Part model, mm, in its own coordinate system. A direction names the side the tool comes from. Round coordinates to 2 decimals unless told otherwise and drop trailing zeros. Loops run counter-clockwise (first coordinate to the right, second up) from the corner with the lowest first, then second, coordinate; pieces in that order, holes last. Notation, with made-up numbers: M -31,24 L 21,24 A17 cw 21,31 Z; hole C -14.5,75.5 d3. An arc over 180 degrees is marked long. Put each result on its own line as item: value. Start each with the question number.
```python
from build123d import *

# Parameters (mm, degrees)
SKETCH_1_W          = 18
SKETCH_1_H          = 5
EXTRUDE_1_DEPTH     = 47.5
SKETCH_2_W          = 24
SKETCH_2_H          = 8
EXTRUDE_2_DEPTH     = 3.5
SKETCH_3_W          = 12.6
SKETCH_3_H          = 2
CUT_EXTRUDE_1_DEPTH = 50.30010142
CHAMFER_1_SIZE      = 1


with BuildPart() as part:
    # 草图1 → 凸台-拉伸1 (new body)
    with BuildSketch(Plane.XY):
        Rectangle(SKETCH_1_W, SKETCH_1_H)
    extrude(amount=EXTRUDE_1_DEPTH)

    # 草图2 → 凸台-拉伸2 (add)
    with BuildSketch(Plane(origin=(0, 0, 0), x_dir=(-1, 0, 0), z_dir=(0, 0, -1))):
        with Locations((0, 1.5)):
            Rectangle(SKETCH_2_W, SKETCH_2_H)
    extrude(amount=-EXTRUDE_2_DEPTH)

    # 草图3 → 切除-拉伸1 (cut, through all)
    with BuildSketch(Plane(origin=(0, 0, 0), x_dir=(-1, 0, 0), z_dir=(0, 0, -1))):
        with Locations((0, -1.5)):
            Rectangle(SKETCH_3_W, SKETCH_3_H)
    extrude(amount=-CUT_EXTRUDE_1_DEPTH, mode=Mode.SUBTRACT)

    # 倒角1
    chamfer_1_edges = [part.edges().sort_by_distance(p)[0] for p in [
        (12, 5.5, 1.75),
        (-12, 5.5, 1.75),
    ]]
    chamfer(chamfer_1_edges, length=CHAMFER_1_SIZE)


solid = part.part
```
1. Cut at B-B, the plane z = 20.5. Give the cut face in (x, y).
2. Which spindle directions (+Z, -Z, +X, -X, +Y, -Y) get a long thin tool onto all of the face, cutting with end or side? Do faces 1 (the flat face through (9, 0, 25)), 2 (the flat face through (0, 2.5, 25)), 3 (the flat face through (-9, 0, 25)), 4 (the flat face through (6.3, -2, 23)). Say none if no direction does.
3. Cut at D-D, the plane x = -8.25. Give the cut face in (y, z), and give its area (3 significant figures).
4. Drop flat-ended pins along their axis: pin 1 (3 mm diameter, centred on x = -5, y = 4.5, fed in from +Z); pin 2 (6.5 mm diameter, centred on x = -0.5, z = 28, fed in from -Y); pin 3 (2.5 mm diameter, centred on y = 1, z = 29, fed in from +X). Give the stop position or say it passes through.
5. Cut at C-C, the plane x = -1. Give the cut face in (y, z), and give its area (3 significant figures).
6. Wall check: L1, parallel to X at y = -1.5, z = 8; L2, parallel to Z at x = -9.25, y = -0.75; L3, parallel to Y at x = 7, z = 38.5. Give the ranges that are in metal, low to high.
7. Cut at A-A, the plane y = 0.5. Give the cut face in (x, z), and give its area (3 significant figures).
Results list:
1. outline: M -9,-2.5 L -6.3,-2.5 L -6.3,-0.5 L 6.3,-0.5 L 6.3,-2.5 L 9,-2.5 L 9,2.5 L -9,2.5 Z
2. face 1: +Z, +X, +Y, -Y
2. face 2: +Z, +X, -X, +Y
2. face 3: +Z, -X, +Y, -Y
2. face 4: +Z, -Z, -Y
3. outline: M -2.5,0 L 5.5,0 L 5.5,3.5 L 2.5,3.5 L 2.5,47.5 L -2.5,47.5 Z
3. area: 248 mm^2
4. pin 1: stops at z = 3.5
4. pin 2: stops at y = -0.5
4. pin 3: stops at x = 9
5. outline: M -0.5,0 L 5.5,0 L 5.5,3.5 L 2.5,3.5 L 2.5,47.5 L -0.5,47.5 Z
5. area: 153 mm^2
6. L1: x = -9 to -6.3, 6.3 to 9
6. L2: z = 0 to 3.5
6. L3: y = -2.5 to 2.5
7. outline: M -12,0 L 12,0 L 12,3.5 L 9,3.5 L 9,47.5 L -9,47.5 L -9,3.5 L -12,3.5 Z
7. area: 876 mm^2
